```python
from build123d import *
from OCP.BRepFilletAPI import BRepFilletAPI_MakeChamfer

# Parameters (mm, degrees)
SKETCH_1_W          = 80
SKETCH_1_H          = 60
SKETCH_1_R          = 2
EXTRUDE_1_DEPTH     = 4
FILLET_1_R          = 5
SKETCH_2_W          = 44
SKETCH_2_H          = 4
SKETCH_2_W_2        = 24
SKETCH_2_H_2        = 4.25
EXTRUDE_2_DEPTH     = 2.5
SKETCH_2_3_W        = 8
SKETCH_2_3_H        = 20
EXTRUDE_3_DEPTH     = 24.5
SKETCH_3_R          = 2
CUT_EXTRUDE_1_DEPTH = 7
CHAMFER_1_SIZE      = 10
CHAMFER_1_SIZE2     = 3.639702343
FILLET_2_R          = 2
FILLET_3_R          = 2


with BuildPart() as part:
    # Эскиз1 → Бобышка-Вытянуть1 (new body)
    with BuildSketch(Plane(origin=(0, 0, 0), x_dir=(1, 0, 0), z_dir=(0, 1, 0))):
        Rectangle(SKETCH_1_W, SKETCH_1_H)
        with Locations(Location((-35, 25, 0), (0, 0, 270))):
            Circle(SKETCH_1_R, mode=Mode.SUBTRACT)
        with Locations(Location((35, 25, 0), (0, 0, 270))):
            Circle(SKETCH_1_R, mode=Mode.SUBTRACT)
        with Locations(Location((-35, -25, 0), (0, 0, 270))):
            Circle(SKETCH_1_R, mode=Mode.SUBTRACT)
        with Locations(Location((35, -25, 0), (0, 0, 270))):
            Circle(SKETCH_1_R, mode=Mode.SUBTRACT)
    extrude(amount=EXTRUDE_1_DEPTH)

    # Скругление1
    fillet_1_edges = [part.edges().sort_by_distance(p)[0] for p in [
        (40, 2, 30),
        (-40, 2, 30),
        (-40, 2, -30),
        (40, 2, -30),
    ]]
    fillet(fillet_1_edges, radius=FILLET_1_R)

    # Эскиз2 → Бобышка-Вытянуть2 (add)
    with BuildSketch(Plane(origin=(0, 4, 0), x_dir=(1, 0, 0), z_dir=(0, 1, 0))):
        with Locations((-3, 28)):
            Rectangle(SKETCH_2_W, SKETCH_2_H)
        with Locations((-13, -8.125)):
            Rectangle(SKETCH_2_W_2, SKETCH_2_H_2)
    extrude(amount=EXTRUDE_2_DEPTH)

    # Эскиз2<3> → Бобышка-Вытянуть3 (add)
    with BuildSketch(Plane(origin=(0, 4, 0), x_dir=(1, 0, 0), z_dir=(0, 1, 0))):
        with Locations((24.5, 10)):
            Rectangle(SKETCH_2_3_W, SKETCH_2_3_H)
        with Locations((-29, 10)):
            Rectangle(SKETCH_2_3_W, SKETCH_2_3_H)
    extrude(amount=EXTRUDE_3_DEPTH)

    # Эскиз3 → Вырез-Вытянуть1 (cut)
    with BuildSketch(Plane(origin=(0, 28.5, 0), x_dir=(1, 0, 0), z_dir=(0, 1, 0))):
        with Locations(Location((-29, 10, 0), (0, 0, 270))):
            Circle(SKETCH_3_R)
        with Locations(Location((24.5, 10, 0), (0, 0, 270))):
            Circle(SKETCH_3_R)
    extrude(amount=-CUT_EXTRUDE_1_DEPTH, mode=Mode.SUBTRACT)

    # Фаска1: one chamfer whose edges measure the first distance from different faces: ONE call of the kernel's chamfer builder (chamfer() names one face for all edges)
    chamfer_1_edges_1 = [part.edges().sort_by_distance(p)[0] for p in [
        (28.5, 4, -10),
    ]]
    chamfer_1_side_1 = [part.faces().sort_by_distance(p)[0] for p in [
        (28.5, 16.25, -10),
    ]]
    chamfer_1_edges_2 = [part.edges().sort_by_distance(p)[0] for p in [
        (-33, 4, -10),
    ]]
    chamfer_1_side_2 = [part.faces().sort_by_distance(p)[0] for p in [
        (-33, 16.25, -10),
    ]]
    chamfer_1 = BRepFilletAPI_MakeChamfer(part.part.solid().wrapped)
    for e in chamfer_1_edges_1:
        chamfer_1.Add(CHAMFER_1_SIZE, CHAMFER_1_SIZE2, e.wrapped, chamfer_1_side_1[0].wrapped)  # the first distance lies on this face
    for e in chamfer_1_edges_2:
        chamfer_1.Add(CHAMFER_1_SIZE, CHAMFER_1_SIZE2, e.wrapped, chamfer_1_side_2[0].wrapped)  # the first distance lies on this face
    add(Compound.cast(chamfer_1.Shape()), mode=Mode.REPLACE)

    # Скругление2
    fillet_2_edges = [part.edges().sort_by_distance(p)[0] for p in [
        (-34.819851171, 9, 0),
        (-34.819851171, 9, -20),
        (30.319851171, 9, 0),
        (30.319851171, 9, -20),
        (28.5, 21.25, -20),
        (20.5, 16.25, -20),
        (20.5, 16.25, 0),
        (28.5, 21.25, 0),
        (-25, 16.25, 0),
        (-25, 16.25, -20),
        (-33, 21.25, -20),
        (-33, 21.25, 0),
    ]]
    fillet(fillet_2_edges, radius=FILLET_2_R)

    # Скругление3
    fillet_3_edges = [part.edges().sort_by_distance(p)[0] for p in [
        (-25, 5.25, -26),
        (19, 5.25, -30),
        (-25, 5.25, -30),
        (19, 5.25, -26),
        (-1, 5.25, 6),
        (-25, 5.25, 6),
        (-25, 5.25, 10.25),
        (-1, 5.25, 10.25),
    ]]
    fillet(fillet_3_edges, radius=FILLET_3_R - 0.0001)  # a hair under: the kernel refuses the full size


solid = part.part
```
Geometry: final body of the model. Coordinates: model frame, mm. A direction names the side the tool comes from. Round coordinates to 2 decimals unless told otherwise and drop trailing zeros. Order: outer loops, then holes, each group sorted by start corner. A loop starts at its lowest first (then second) coordinate and runs counter-clockwise, first axis right, second up. Notation, with made-up numbers: (40.5, 45) -> (52.5, 45) arc R18 cw to (52.5, 63) -> close; hole circle Ø8 at (8, 74). An arc over 180 degrees is marked (long way). Use one line per item in the form item = value. Start each with the question number.
1. Draft query along X for faces 6 (the face through (24.4, 28.5, -12.4)), 7 (the face through (27.93, 21.18, -19.4)), 8 (the face through (-29, 21.5, -10)), 9 (the face through (-34.845, 8.93, -9.888)). Return one class per face: pulls with the +X half, pulls with the -X half, needs draft (parallel to the pull), parting line crosses it, or undercut.
2. Cut plane B-B (x = -15.5). Return the cut outline in (y, z), then the cut area to 3 significant figures.
3. Reachability of faces 1 (the face through (-1.6, 5.27, 6.57)), 2 (the face through (21.07, 16.42, -0.6)), 3 (the face through (-32.43, 21.18, -19.4)), 4 (the face through (-24.43, 5.27, 6.6)), 5 (the face through (25, 16, -20)) from +Z, -Z, +X, -X, +Y, -Y: full face, straight path, thin tool, end or side. Return the list, or none.
4. Pin query (flat end, axial travel): pin 1 Ø3.5 at (x, z) = (35, -25) entering from +Y; pin 2 Ø5 at (x, y) = (-28, 23) entering from -Z; pin 3 Ø1 at (x, z) = (-4, -6) entering from +Y; pin 4 Ø6 at (x, y) = (27, 11) entering from +Z. Return the tip coordinate at first contact, or that it passes through.
5. Cut plane A-A (y = 24.5). Return the cut outline in (x, z), then the cut area to 3 significant figures.
6. Line query: probe 1 along X at (y, z) = (1, 25); probe 2 along X at (y, z) = (27.25, -10); probe 3 along Y at (x, z) = (-27, 8.5). Output: solid intervals per line, ascending.
7. Cut plane C-C (y = 18). Return the cut outline in (x, z), then the cut area to 3 significant figures.
8. Cut plane D-D (z = -17). Return the cut outline in (x, y), then the cut area to 3 significant figures.
Solution:
q1.face_6 = needs draft
q1.face_7 = pulls with the +X half
q1.face_8 = undercut
q1.face_9 = pulls with the -X half
q2.outline = (0, -30) -> (6.5, -30) -> (6.5, -26) -> (4, -26) -> (4, 6) -> (6.5, 6) -> (6.5, 10.25) -> (4, 10.25) -> (4, 30) -> (0, 30) -> close
q2.area = 261 mm^2
q3.face_1 = +X, +Y
q3.face_2 = +Z, +Y
q3.face_3 = -Z, -X, +Y
q3.face_4 = -X, +Y
q3.face_5 = -Z, +X, -X, +Y
q4.pin_1 = through
q4.pin_2 = -20
q4.pin_3 = 4
q4.pin_4 = 0
q5.outline = (-33, -18) arc R2 ccw to (-31, -20) -> (-27, -20) arc R2 ccw to (-25, -18) -> (-25, -2) arc R2 ccw to (-27, 0) -> (-31, 0) arc R2 ccw to (-33, -2) -> close; (20.5, -18) arc R2 ccw to (22.5, -20) -> (26.5, -20) arc R2 ccw to (28.5, -18) -> (28.5, -2) arc R2 ccw to (26.5, 0) -> (22.5, 0) arc R2 ccw to (20.5, -2) -> close; hole circle Ø4 at (-29, -10); hole circle Ø4 at (24.5, -10)
q5.area = 288 mm^2
q6.probe_1 = -40 to -37, -33 to 33, 37 to 40
q6.probe_2 = -33 to -31, -27 to -25, 20.5 to 22.5, 26.5 to 28.5
q6.probe_3 = 0 to 4
q7.outline = (-33, -18) arc R2 ccw to (-31, -20) -> (-27, -20) arc R2 ccw to (-25, -18) -> (-25, -2) arc R2 ccw to (-27, 0) -> (-31, 0) arc R2 ccw to (-33, -2) -> close; (20.5, -18) arc R2 ccw to (22.5, -20) -> (26.5, -20) arc R2 ccw to (28.5, -18) -> (28.5, -2) arc R2 ccw to (26.5, 0) -> (22.5, 0) arc R2 ccw to (20.5, -2) -> close
q7.area = 313 mm^2
q8.outline = (-40, 0) -> (40, 0) -> (40, 4) -> (32.14, 4) -> (28.5, 14) -> (28.5, 28.5) -> (20.5, 28.5) -> (20.5, 4) -> (-25, 4) -> (-25, 28.5) -> (-33, 28.5) -> (-33, 14) -> (-36.64, 4) -> (-40, 4) -> close
q8.area = 748 mm^2
